```python
from build123d import *

# Parameters (mm, degrees)
SKETCH1_W           = 7
SKETCH1_H           = 3.2
BOSS_EXTRUDE1_DEPTH = 11.7


with BuildPart() as part:
    # Sketch1 → Boss-Extrude1 (new body)
    with BuildSketch(Plane(origin=(0, 0, 0), x_dir=(0, 0, -1), z_dir=(1, 0, 0))):
        Rectangle(SKETCH1_W, SKETCH1_H)
        Polygon((3.5, 1.6), (3.5, -1.6), (3.5, -11.404255319), (7.393617021, -11.404255319), (7.393617021, 1.6), align=None)
    extrude(amount=BOSS_EXTRUDE1_DEPTH)


solid = part.part
```
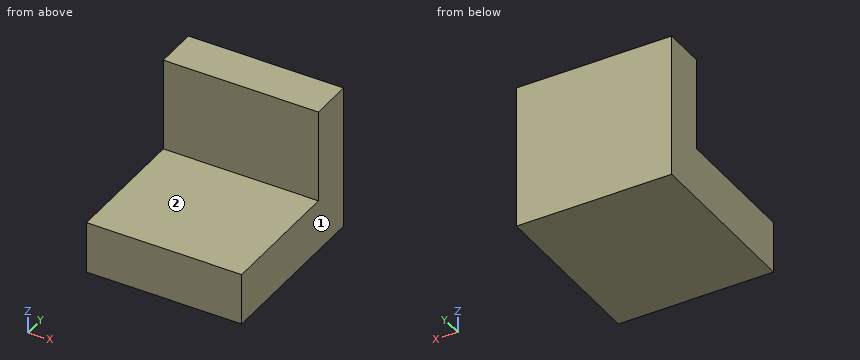
Part model, mm, in its own coordinate system. Face numbers are marked on the shaded views. A direction names the side the tool comes from. Round coordinates to 2 decimals unless told otherwise and drop trailing zeros. Loops run counter-clockwise (first coordinate to the right, second up) from the corner with the lowest first, then second, coordinate; pieces in that order, holes last. Notation, with made-up numbers: (88, -31.5) -> (94, -31.5) arc R27 ccw to (94, 7.5) -> close; hole circle Ø10 at (-4.75, -25.5). An arc over 180 degrees is marked (long way). Use CSV: the item, a comma, the result in double quotes. Start each with the question number.
1) Cut at B-B, the plane y = -3.25. Write the cut outline in (x, z), plus the area to 3 significant figures.
2) Wall check: L1, parallel to Z at x = 2.5, y = -2.5; L2, parallel to Y at x = 8.25, z = 2.5. Give the ranges that are in metal, low to high. Write a range as [from, to].
3) Cut at C-C, the plane z = 1.25. Write the cut outline in (x, y), plus the area to 3 significant figures.
4) Drop flat-ended pins along their axis: P1, Ø3, axis at x = 6, y = -8, coming from the +Z side; P2, Ø2, axis at x = 8, z = 0.5, coming from the -Y side. Give the stop position or say it passes through.
5) Cut at A-A, the plane x = 7.5. Write the cut outline in (y, z).
6) Which spindle directions (+Z, -Z, +X, -X, +Y, -Y) get a long thin tool onto all of the face, cutting with end or side? Do the marked faces 1 and 2. Say none if no direction does.
Determined:
1,outline,"(0, -7.39) -> (11.7, -7.39) -> (11.7, -3.5) -> (0, -3.5) -> close"
1,area,"45.6 mm2"
2,L1,"z = [-7.39, -3.5]"
2,L2,"y = [-1.6, 1.6]"
3,outline,"(0, -1.6) -> (11.7, -1.6) -> (11.7, 1.6) -> (0, 1.6) -> close"
3,area,"37.4 mm2"
4,P1,"stops at z = -3.5"
4,P2,"stops at y = -1.6"
5,outline,"(-11.4, -7.39) -> (1.6, -7.39) -> (1.6, 3.5) -> (-1.6, 3.5) -> (-1.6, -3.5) -> (-11.4, -3.5) -> close"
6,face 1,"+Z, -Z, +X, +Y, -Y"
6,face 2,"+Z, +X, -X, -Y"
